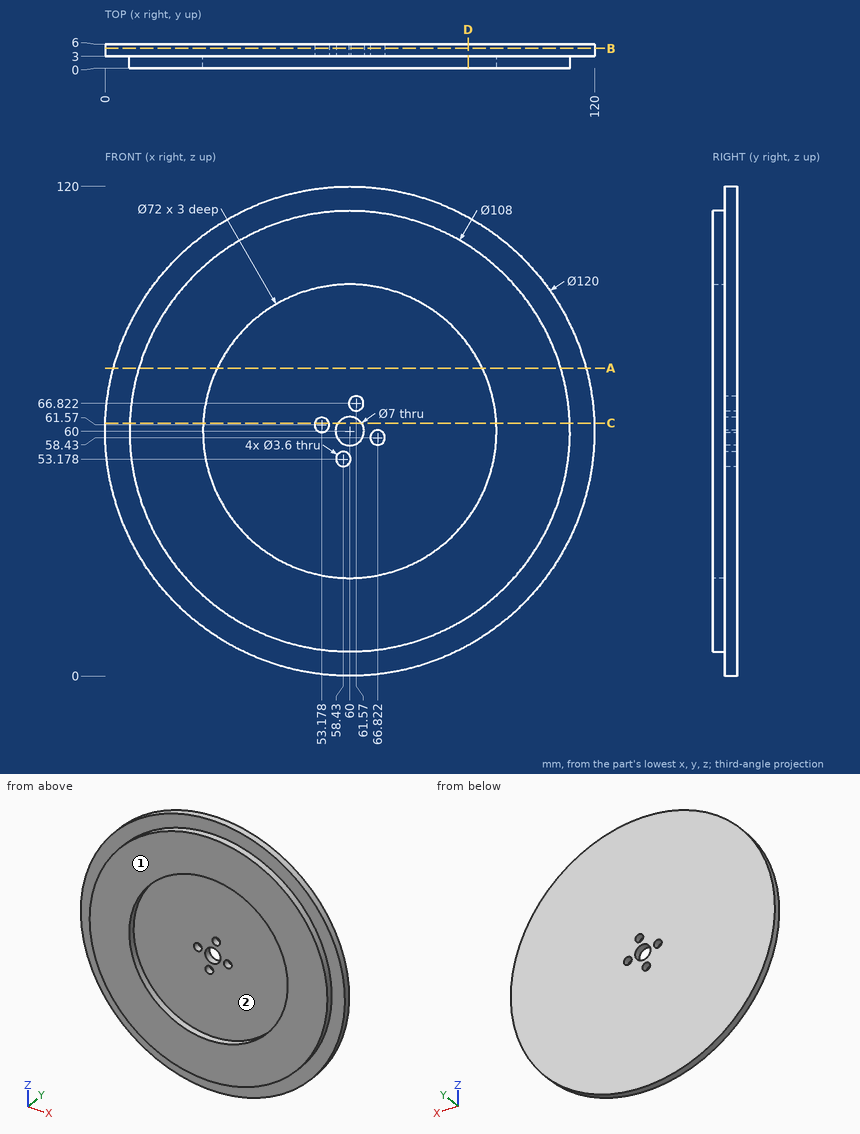
Could you check a few things on this drawing? It's one solid part, dimensions in mm from its lowest x, y, z. Give positions to 0.01 mm unless a question says otherwise; leave off trailing zeros. Order: outer loops, then holes, each group sorted by start corner. A loop starts at its lowest first (then second) coordinate and runs counter-clockwise, first axis right, second up. Notation, with made-up numbers: (60.25, 73.5) -> (71.25, 73.5) arc R14 ccw to (71.25, 96.5) -> close; hole circle Ø6 at (49.25, 79.25). An arc over 180 degrees is marked (long way). Answer in a Markdown table with one row per item. Add a question column.
Item 1: Imagine slicing it at B-B (y = 4.9). List the corners of the cut face in (x, z) for me, and give its area (3 significant figures).
Item 2: Please list where these lines run through material, in increasing order: probe 1 along X at (y, z) = (4.8, 59) (1 decimal); probe 2 along X at (y, z) = (2.85, 35.5); probe 3 along X at (y, z) = (4.3, 60) (1 decimal).
Item 3: Imagine slicing it at A-A (z = 75.5). List the corners of the cut face in (x, y) for me.
Item 4: We'd pull the mould along X, two halves only. Please class the marked faces 1 and 2: pulls with the +X half, pulls with the -X half, needs draft (parallel to the pull), parting line crosses it, or undercut.
Item 5: Imagine slicing it at D-D (x = 89). List the corners of the cut face in (y, z) for me.
Item 6: I'm going to push flat-ended pins straight in: P1, Ø1.5, axis at y = 2, z = 20, coming from the +X side; P2, Ø5.5, axis at x = 60, z = 60, coming from the -Y side; P3, Ø2, axis at x = 18, y = 3.5, coming from the -Z side; P4, Ø6, axis at x = 58.43, z = 53.18, coming from the -Y side. Where does each tip first touch, or does it pass through?
Item 7: Imagine slicing it at C-C (z = 62). List the corners of the cut face in (x, y) for me (1 decimal), and give its area (3 significant figures).
Result:
| question | item | result |
|---|---|---|
| 1 | outline | circle Ø120 at (60, 60); hole circle Ø3.6 at (53.18, 61.57); hole circle Ø7 at (60, 60); hole circle Ø3.6 at (58.43, 53.18); hole circle Ø3.6 at (61.57, 66.82); hole circle Ø3.6 at (66.82, 58.43) |
| 1 | area | 11,200 mm2 |
| 2 | probe 1 | 0 to 56.6, 63.4 to 65.1, 68.5 to 120 |
| 2 | probe 2 | 11.88 to 33.62, 86.38 to 108.12 |
| 2 | probe 3 | 0 to 52.3, 54.1 to 56.5, 63.5 to 65.9, 67.7 to 120 |
| 3 | outline | (2.04, 3) -> (8.27, 3) -> (8.27, 0) -> (27.51, 0) -> (27.51, 3) -> (92.49, 3) -> (92.49, 0) -> (111.73, 0) -> (111.73, 3) -> (117.96, 3) -> (117.96, 6) -> (2.04, 6) -> close |
| 4 | face 1 | needs draft |
| 4 | face 2 | undercut |
| 5 | outline | (0, 14.45) -> (3, 14.45) -> (3, 7.47) -> (6, 7.47) -> (6, 112.53) -> (3, 112.53) -> (3, 105.55) -> (0, 105.55) -> (0, 81.33) -> (3, 81.33) -> (3, 38.67) -> (0, 38.67) -> close |
| 6 | P1 | x = 97.09 |
| 6 | P2 | through |
| 6 | P3 | z = 16.19 |
| 6 | P4 | y = 3 |
| 7 | outline | (0, 3) -> (6, 3) -> (6, 0) -> (24.1, 0) -> (24.1, 3) -> (51.4, 3) -> (51.4, 6) -> (0, 6) -> close; (54.9, 3) -> (57.1, 3) -> (57.1, 6) -> (54.9, 6) -> close; (62.9, 3) -> (95.9, 3) -> (95.9, 0) -> (114, 0) -> (114, 3) -> (120, 3) -> (120, 6) -> (62.9, 6) -> close |
| 7 | area | 440 mm2 |
